Verification items for this drawing (mm, ordinates from the low corner). A direction names the side the tool comes from. Coordinates: 2 decimals unless noted, no trailing zeros. Write each loop counter-clockwise with the first axis right and the second up, starting at its lowest first coordinate (ties: lowest second). Pieces come first, ordered by that corner, then holes. Notation, with made-up numbers: (77.25, 18.5) -> (128.25, 18.5) arc R8 cw to (128.25, 27.5) -> close; hole circle Ø1 at (15, 17). An arc over 180 degrees is marked (long way). One line per item, written item: value. Start each with the question number.
1) Set-up check for the marked faces 1 and 2: record each of +Z, -Z, +X, -X, +Y, -Y from which the full face is reachable in a straight line by a thin tool's end or side.
2) Scan lines: line 1 along Z through (x, y) = (34.5, 13); line 2 along Y through (x, z) = (14.5, 40); line 3 along X through (y, z) = (7.25, 32). Record each from-to range of solid material in increasing order. Write a range as [from, to].
3) Sectioned sample at B-B on x = 34.5. Enter the section's corners in (y, z).
4) Gauge pin test, flat ends, axial feed: P1, Ø14.5, axis at x = 6, z = 64, coming from the -Y side; P2, Ø4.5, axis at y = 6.5, z = 72.5, coming from the -X side. Record the tip position at first contact, or that the pin passes through.
5) Sectioned sample at A-A on z = 15. Enter the section's corners in (x, y), plus the area to 3 significant figures.
6) Sectioned sample at C-C on y = 5. Enter the section's corners in (x, z).
7) Sectioned sample at D-D on x = 6. Enter the section's corners in (y, z), plus the area to 3 significant figures.
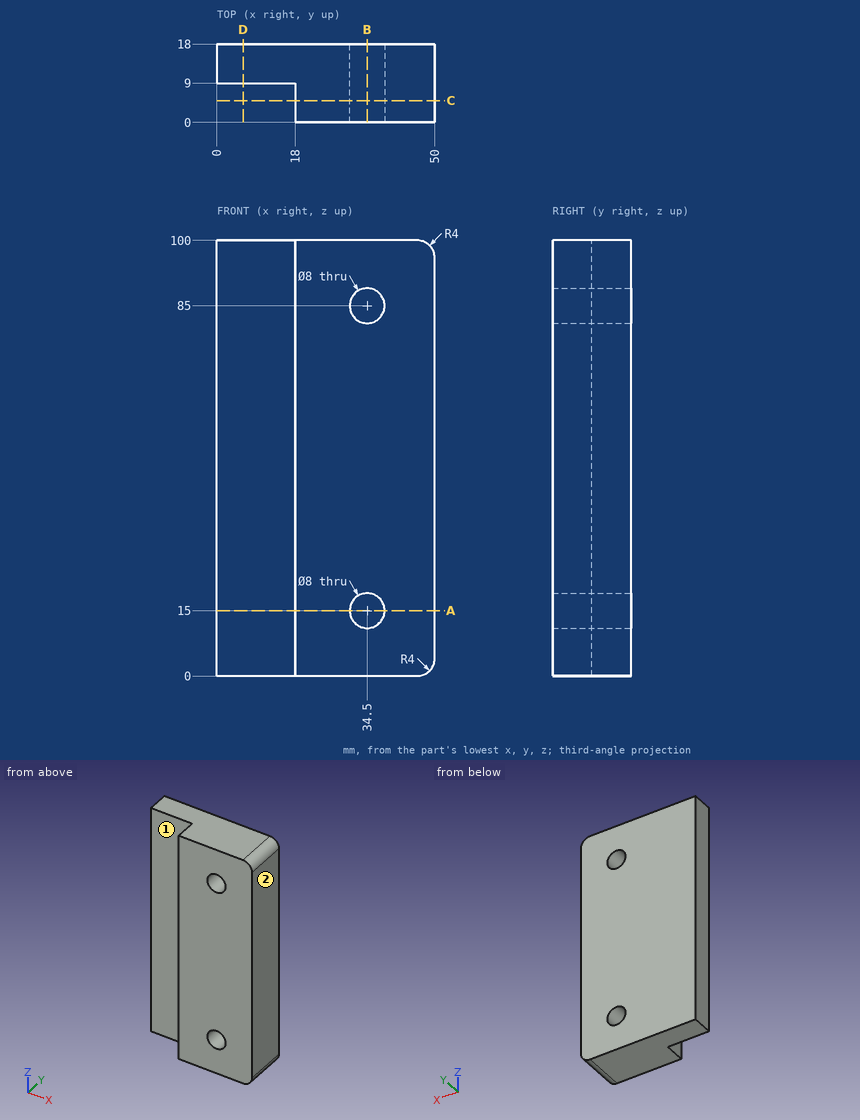
Answers:
1. face 1: +Z, -Z, -X, -Y
1. face 2: +Z, -Z, +X, +Y, -Y
2. line 1: z = [0, 11], [19, 81], [89, 100]
2. line 2: y = [9, 18]
2. line 3: x = [18, 50]
3. outline: (0, 0) -> (18, 0) -> (18, 11) -> (0, 11) -> close; (0, 19) -> (18, 19) -> (18, 81) -> (0, 81) -> close; (0, 89) -> (18, 89) -> (18, 100) -> (0, 100) -> close
4. P1: stops at y = 9
4. P2: stops at x = 18
5. outline: (0, 9) -> (18, 9) -> (18, 0) -> (30.5, 0) -> (30.5, 18) -> (0, 18) -> close; (38.5, 0) -> (50, 0) -> (50, 18) -> (38.5, 18) -> close
5. area: 594 mm2
6. outline: (18, 0) -> (46, 0) arc R4 ccw to (50, 4) -> (50, 96) arc R4 ccw to (46, 100) -> (18, 100) -> close; hole circle Ø8 at (34.5, 15); hole circle Ø8 at (34.5, 85)
7. outline: (9, 0) -> (18, 0) -> (18, 100) -> (9, 100) -> close
7. area: 900 mm2
